Build history of the part. All positions in model axes, mm. Give positions to 0.01 mm unless a question says otherwise; leave off trailing zeros. Write each loop counter-clockwise with the first axis right and the second up, starting at its lowest first coordinate (ties: lowest second). Pieces come first, ordered by that corner, then holes. Notation, with made-up numbers: (70, 19.25) -> (82, 19.25) arc R31 cw to (82, 50.25) -> close; hole circle Ø9 at (88, -26). An arc over 180 degrees is marked (long way). One line per question, with ' | ' between items. Start each with the question number.
(1) Band-saw the part on B-B, the plane y = 673. Give the cut face in (x, z), and give its area (3 significant figures).
(2) Drill centre lines: probe 1 along X at (y, z) = (625, 5.5); probe 2 along X at (y, z) = (605, 3.5); probe 3 along X at (y, z) = (516, 0.5). Where is each one in solid material? Low to high. Write a range as from..to.
(3) Pull direction X, two halves, no side cores. Call faces 1 (the flat face through (23.14, 243.85, 4.93)), 2 (the flat face through (31, 352, 10)): released by +X, released by -X, zero draft, split by the parting line, or undercut.
(4) Band-saw the part on A-A, the plane z = 2. Count the separate pieces of the cut face and the enclosed holes in it, and give its area (3 significant figures).
from build123d import *

# Parameters (mm, degrees)
ESQUISSE1_W                  = 50
ESQUISSE1_H                  = 594
BOSS_EXTRU_1_DEPTH           = 10
ENL_V_MAT_EXTRU_1_DEPTH      = 597.18453519
ENL_V_MAT_EXTRU_1_DEPTH_BACK = 597.18453519
CONG_1_R                     = 4
ESQUISSE3_W                  = 50
ESQUISSE3_H                  = 30
BOSS_EXTRU_2_DEPTH           = 10
ENL_V_MAT_EXTRU_2_DEPTH      = 597.18453519
ENL_V_MAT_EXTRU_2_DEPTH_BACK = 597.18453519
ESQUISSE4_R                  = 3
BOSS_EXTRU_3_DEPTH           = 10
ENL_V_MAT_EXTRU_3_DEPTH      = 726.793359022
ENL_V_MAT_EXTRU_3_DEPTH_BACK = 726.793359022
ESQUISSE6_R                  = 4
ESQUISSE6_R_2                = 5
CONG_2_R                     = 5
CONG_3_R                     = 20


with BuildPart() as part:
    # Esquisse1 → Boss.-Extru.1 (new body)
    with BuildSketch(Plane.XY):
        with Locations((25, 297)):
            Rectangle(ESQUISSE1_W, ESQUISSE1_H)
    extrude(amount=BOSS_EXTRU_1_DEPTH)

    # Esquisse2 → Enlèv. mat.-Extru.1 (cut, two sides: drawn at the far end of the back side and taken through both)
    with BuildSketch(Plane.XY.offset(10).offset(-ENL_V_MAT_EXTRU_1_DEPTH_BACK)):
        Polygon((10, 10), (40, 10), (10, 40), align=None)
        Polygon((40, 24.142135624), (10, 54.142135624), (40, 84.142135624), align=None)
        Polygon((10, 68.284271247), (10, 128.284271247), (40, 98.284271247), align=None)
        Polygon((40, 172.426406871), (10, 142.426406871), (40, 112.426406871), align=None)
        Polygon((10, 156.568542495), (10, 216.568542495), (40, 186.568542495), align=None)
        Polygon((40, 260.710678119), (10, 230.710678119), (40, 200.710678119), align=None)
        Polygon((40, 274.852813742), (10, 244.852813742), (10, 274.852813742), align=None)
        Polygon((40, 348.994949366), (10, 318.994949366), (40, 318.994949366), align=None)
        Polygon((10, 333.13708499), (10, 393.13708499), (40, 363.13708499), align=None)
        Polygon((40, 437.279220614), (10, 407.279220614), (40, 377.279220614), align=None)
        Polygon((10, 421.421356237), (10, 481.421356237), (40, 451.421356237), align=None)
        Polygon((40, 525.563491861), (10, 495.563491861), (40, 465.563491861), align=None)
        Polygon((10, 509.705627485), (10, 569.705627485), (40, 539.705627485), align=None)
        Polygon((10, 583.847763109), (40, 553.847763109), (40, 583.847763109), align=None)
    extrude(amount=ENL_V_MAT_EXTRU_1_DEPTH + ENL_V_MAT_EXTRU_1_DEPTH_BACK, mode=Mode.SUBTRACT)

    # Congé1
    cong_1_edges = [part.edges().sort_by_distance(p)[0] for p in [
        (40, 112.426406871, 5),
        (10, 142.426406871, 5),
        (40, 172.426406871, 5),
        (40, 539.705627485, 5),
        (10, 509.705627485, 5),
        (10, 569.705627485, 5),
        (40, 377.279220614, 5),
        (10, 407.279220614, 5),
        (40, 437.279220614, 5),
        (40, 363.13708499, 5),
        (10, 333.13708499, 5),
        (10, 393.13708499, 5),
        (40, 465.563491861, 5),
        (10, 495.563491861, 5),
        (40, 525.563491861, 5),
        (40, 451.421356237, 5),
        (10, 421.421356237, 5),
        (10, 481.421356237, 5),
        (10, 10, 5),
        (10, 40, 5),
        (40, 10, 5),
        (40, 200.710678119, 5),
        (10, 230.710678119, 5),
        (40, 260.710678119, 5),
        (40, 186.568542495, 5),
        (10, 156.568542495, 5),
        (10, 216.568542495, 5),
        (10, 244.852813742, 5),
        (10, 274.852813742, 5),
        (40, 274.852813742, 5),
        (40, 318.994949366, 5),
        (10, 318.994949366, 5),
        (40, 348.994949366, 5),
        (40, 98.284271247, 5),
        (10, 68.284271247, 5),
        (10, 128.284271247, 5),
        (40, 84.142135624, 5),
        (40, 24.142135624, 5),
        (10, 54.142135624, 5),
        (10, 583.847763109, 5),
        (40, 583.847763109, 5),
        (40, 553.847763109, 5),
    ]]
    fillet(cong_1_edges, radius=CONG_1_R)

    # Esquisse3 → Boss.-Extru.2 (add)
    with BuildSketch(Plane.XY.offset(10)):
        with Locations((25, -15)):
            Rectangle(ESQUISSE3_W, ESQUISSE3_H)
    extrude(amount=-BOSS_EXTRU_2_DEPTH)

    # Esquisse4 → Enlèv. mat.-Extru.2 (cut, two sides: drawn at the far end of the back side and taken through both)
    with BuildSketch(Plane.XY.offset(10).offset(-ENL_V_MAT_EXTRU_2_DEPTH_BACK)):
        with Locations((39, 296.923881554)):
            Circle(ESQUISSE4_R)
        with Locations(Location((11, 296.923881554, 0), (0, 0, 180))):
            Circle(ESQUISSE4_R)
    extrude(amount=ENL_V_MAT_EXTRU_2_DEPTH + ENL_V_MAT_EXTRU_2_DEPTH_BACK, mode=Mode.SUBTRACT)

    # Esquisse5 → Boss.-Extru.3 (add)
    with BuildSketch(Plane.XY.offset(10)):
        Polygon((50, 594), (0, 594), (0, 724), (24.522083601, 724), (50, 654), align=None)
    extrude(amount=-BOSS_EXTRU_3_DEPTH)

    # Esquisse6 → Enlèv. mat.-Extru.3 (cut, two sides: drawn at the far end of the back side and taken through both)
    with BuildSketch(Plane(origin=(0, 0, 0), x_dir=(-1, 0, 0), z_dir=(0, 0, -1)).offset(-ENL_V_MAT_EXTRU_3_DEPTH_BACK)):
        with Locations((-15, 625)):
            Circle(ESQUISSE6_R)
        with Locations((-35, 605)):
            Circle(ESQUISSE6_R)
        with Locations((-20, 685)):
            Circle(ESQUISSE6_R_2)
    extrude(amount=ENL_V_MAT_EXTRU_3_DEPTH + ENL_V_MAT_EXTRU_3_DEPTH_BACK, mode=Mode.SUBTRACT)

    # Congé2
    cong_2_edges = [part.edges().sort_by_distance(p)[0] for p in [
        (0, 724, 5),
        (24.522083601, 724, 5),
    ]]
    fillet(cong_2_edges, radius=CONG_2_R)

    # Congé3
    cong_3_edges = [part.edges().sort_by_distance(p)[0] for p in [
        (50, 654, 5),
    ]]
    fillet(cong_3_edges, radius=CONG_3_R)


solid = part.part
Results:
1) outline: (0, 0) -> (43.08, 0) -> (43.08, 10) -> (0, 10) -> close | area: 431 mm²
2) probe 1: x = 0..11, 19..50 | probe 2: x = 0..31, 39..50 | probe 3: x = 0..11.83, 16.17..30.44, 40..50
3) face 1: undercut | face 2: zero draft
4) separate pieces: 1 | enclosed holes: 19 | area: 26,400 mm²
